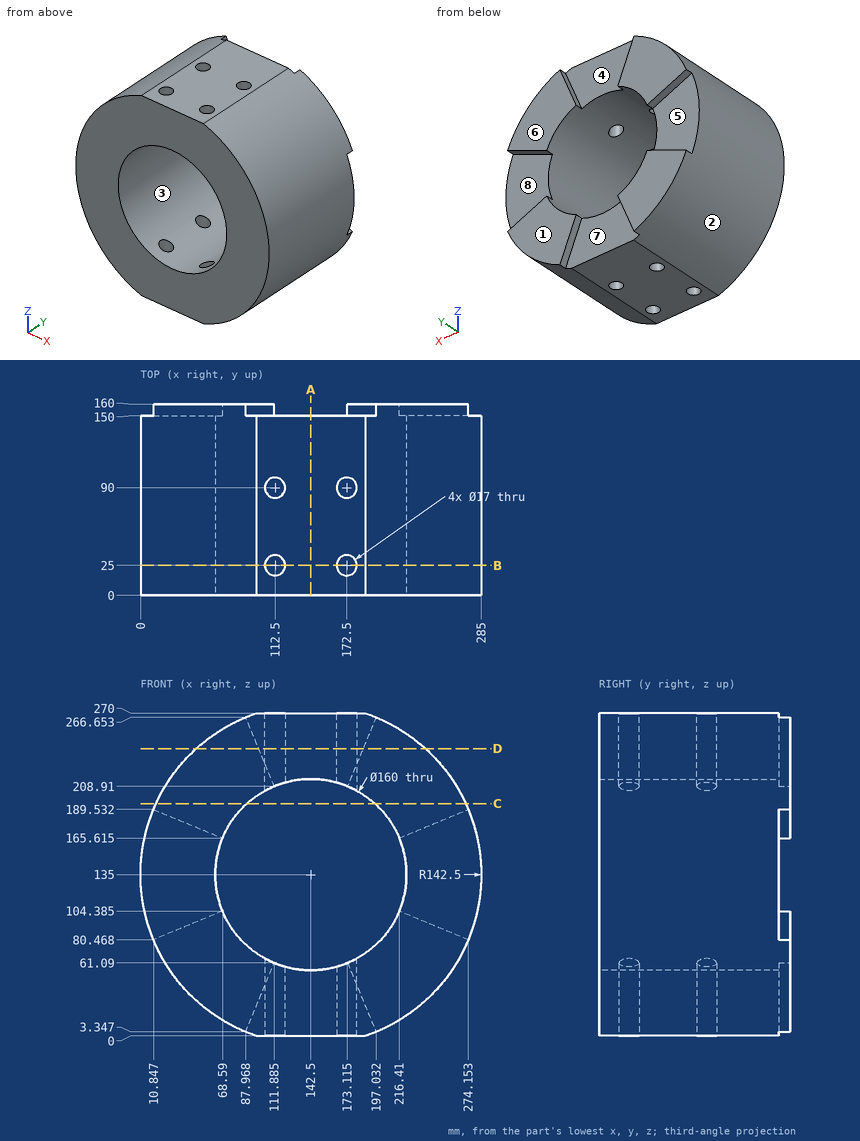
The drawing under review shows one solid part. Ordinate dimensions are in mm from its lowest x, y, z. A direction names the side the tool comes from. Coordinates: 2 decimals unless noted, no trailing zeros. Order: outer loops, then holes, each group sorted by start corner. A loop starts at its lowest first (then second) coordinate and runs counter-clockwise, first axis right, second up. Notation, with made-up numbers: (80, 73.5) -> (126, 73.5) arc R18 ccw to (126, 108.5) -> close; hole circle Ø2 at (50, 23.5). An arc over 180 degrees is marked (long way). Answer as CSV lines item,"result".
Q1. We need section D-D (z = 240.5). State the section outline as (x, y) points.
Model answer:
outline,"(46.71, 0) -> (238.29, 0) -> (238.29, 160) -> (186.2, 160) -> (186.2, 150) -> (98.8, 150) -> (98.8, 160) -> (46.71, 160) -> close; hole circle Ø17 at (112.5, 25); hole circle Ø17 at (112.5, 90); hole circle Ø17 at (172.5, 25); hole circle Ø17 at (172.5, 90)"
Q2. Draft analysis for pull direction X (two halves, no side actions). For the marked faces 1, 2 and 3, state which applies: released by +X, released by -X, zero draft, split by the parting line, or undercut.
Model answer:
face 1,"zero draft"
face 2,"released by -X"
face 3,"undercut"
Q3. For the marked faces 4, 5, 6, 7 and 8, list the 3-axis set-ups (+Z, -Z, +X, -X, +Y, -Y) from which the entire face can be reached by the end or side of a thin tool; tool diameter is ignored.
Model answer:
face 4,"+Z, +Y"
face 5,"-X, +Y"
face 6,"+Z, -Z, +X, -X, +Y"
face 7,"-Z, +Y"
face 8,"+X, +Y"
Q4. We need section C-C (z = 194.5). State the section outline as (x, y) points.
Model answer:
outline,"(13.02, 0) -> (89.02, 0) -> (89.02, 160) -> (13.02, 160) -> close; (195.98, 0) -> (271.98, 0) -> (271.98, 160) -> (195.98, 160) -> close"
Q5. We need section B-B (y = 25). State the section outline as (x, z) points.
Model answer:
outline,"(96.88, 0) -> (104, 0) -> (104, 64.87) arc R80 cw to (104, 205.13) -> (104, 270) -> (96.88, 270) arc R142.5 ccw to start; (121, 0) -> (164, 0) -> (164, 57.94) arc R80 cw to (121, 57.94) -> close; (121, 212.06) arc R80 cw to (164, 212.06) -> (164, 270) -> (121, 270) -> close; (181, 0) -> (188.12, 0) arc R142.5 ccw to (188.12, 270) -> (181, 270) -> (181, 205.13) arc R80 cw to (181, 64.87) -> close"
Q6. Clearance check with flat-ended pins moving along their axes: pin 1 Ø3 at (y, z) = (66, 84) entering from -X; pin 2 Ø10 at (x, y) = (229.5, 110) entering from -Z; pin 3 Ø20.5 at (x, z) = (246.5, 121) entering from +Y; pin 4 Ø15.5 at (x, y) = (172.5, 25) entering from -Z. State where each tip first meets the part, or that it passes through.
Model answer:
pin 1,"stops at x = 8.87"
pin 2,"stops at z = 18.46"
pin 3,"stops at y = 150"
pin 4,"passes through"
Q7. We need section A-A (x = 142.5). State the section outline as (y, z) points.
Model answer:
outline,"(0, 0) -> (150, 0) -> (150, 55) -> (0, 55) -> close; (0, 215) -> (150, 215) -> (150, 270) -> (0, 270) -> close"
Q8. Wall thickness on line 1 along Y through (x, z) = (172, 244) (1 decimal); line 2 along Z through (x, y) = (142.5, 82); line 3 along X through (y, z) = (84, 135): over which ranges is each line inside the solid? List them lowest first. Write a range as [from, to].
Model answer:
line 1,"y = [0, 16.5], [33.5, 81.5], [98.5, 150]"
line 2,"z = [0, 55], [215, 270]"
line 3,"x = [0, 62.5], [222.5, 285]"
